from build123d import *

# Parameters (mm, degrees)
SKETCH_1_R      = 30
EXTRUDE_1_DEPTH = 20


with BuildPart() as part:
    # 草图1 → 凸台-拉伸1 (new body)
    with BuildSketch(Plane.XY):
        Circle(SKETCH_1_R)
        with BuildLine():
            Line((-3.088645972, 2.69634309), (-2.908227328, -2.89001969))
            ThreePointArc((-2.908227328, -2.89001969), (4.097863422, 0.132345676), (-3.088645972, 2.69634309))
        make_face(mode=Mode.SUBTRACT)
        with BuildLine():
            Line((22.596573624, 14.778188672), (6.935213074, 5.736097943))
            ThreePointArc((6.935213074, 5.736097943), (4.5, 7.794228634), (1.5, 8.874119675))
            Line((1.5, 8.874119675), (1.5, 26.958301133))
            ThreePointArc((1.5, 26.958301133), (13.5, 23.382685902), (22.596573624, 14.778188672))
        make_face(mode=Mode.SUBTRACT)
        with BuildLine():
            Line((-1.5, 26.958301133), (-1.5, 8.874119675))
            ThreePointArc((-1.5, 8.874119675), (-4.5, 7.794228634), (-6.935213074, 5.736097943))
            Line((-6.935213074, 5.736097943), (-22.596573624, 14.778188672))
            ThreePointArc((-22.596573624, 14.778188672), (-13.5, 23.382685902), (-1.5, 26.958301133))
        make_face(mode=Mode.SUBTRACT)
        with BuildLine():
            Line((24.096573624, 12.180112461), (8.435213074, 3.138021732))
            ThreePointArc((8.435213074, 3.138021732), (9, 0), (8.435213074, -3.138021732))
            Line((8.435213074, -3.138021732), (24.096573624, -12.180112461))
            ThreePointArc((24.096573624, -12.180112461), (27, 0), (24.096573624, 12.180112461))
        make_face(mode=Mode.SUBTRACT)
        with BuildLine():
            Line((22.596573624, -14.778188672), (6.935213074, -5.736097943))
            ThreePointArc((6.935213074, -5.736097943), (4.5, -7.794228634), (1.5, -8.874119675))
            Line((1.5, -8.874119675), (1.5, -26.958301133))
            ThreePointArc((1.5, -26.958301133), (13.5, -23.382685902), (22.596573624, -14.778188672))
        make_face(mode=Mode.SUBTRACT)
        with BuildLine():
            Line((-1.5, -26.958301133), (-1.5, -8.874119675))
            ThreePointArc((-1.5, -8.874119675), (-4.5, -7.794228634), (-6.935213074, -5.736097943))
            Line((-6.935213074, -5.736097943), (-22.596573624, -14.778188672))
            ThreePointArc((-22.596573624, -14.778188672), (-13.5, -23.382685902), (-1.5, -26.958301133))
        make_face(mode=Mode.SUBTRACT)
        with BuildLine():
            Line((-24.096573624, -12.180112461), (-8.435213074, -3.138021732))
            ThreePointArc((-8.435213074, -3.138021732), (-9, 0), (-8.435213074, 3.138021732))
            Line((-8.435213074, 3.138021732), (-24.096573624, 12.180112461))
            ThreePointArc((-24.096573624, 12.180112461), (-27, 0), (-24.096573624, -12.180112461))
        make_face(mode=Mode.SUBTRACT)
    extrude(amount=EXTRUDE_1_DEPTH)

    # 草图2 → 旋转1 (revolve)
    with BuildSketch(Plane.ZY, mode=Mode.PRIVATE) as revolve_1_sk:
        Polygon((0, -30), (0, -33), (1.6, -33), (3, -30), align=None)
        Polygon((17, -30), (20, -30), (20, -33), (18.4, -33), align=None)
        Polygon((7.8, -30), (9.2, -33), (10.8, -33), (12.2, -30), align=None)
    revolve(revolve_1_sk.sketch.rotate(Axis((0, 0, 0), (0, 0, 1)), 270), axis=Axis((0, 0, 0), (0, 0, 1)))


solid = part.part
Geometry check sheet. Reference: the model listing, model coordinates, mm. A direction names the side the tool comes from. Give positions to 0.01 mm unless a question says otherwise; leave off trailing zeros. Order: outer loops, then holes, each group sorted by start corner. A loop starts at its lowest first (then second) coordinate and runs counter-clockwise, first axis right, second up. Notation, with made-up numbers: M 88.5,24 L 116.5,24 A18 cw 116.5,45 Z; hole C -25.75,11.5 d8. An arc over 180 degrees is marked long. Use a Markdown table: item, result.
Item 1: Section check B-B (x = 0). Record the cut outline in (y, z).
Answers follow:
| item | result |
|---|---|
| outline | M -33,0 L -4.1,0 L -4.1,20 L -33,20 L -33,18.4 L -30,17 L -30,12.2 L -33,10.8 L -33,9.2 L -30,7.8 L -30,3 L -33,1.6 Z; M 4.1,0 L 33,0 L 33,1.6 L 30,3 L 30,7.8 L 33,9.2 L 33,10.8 L 30,12.2 L 30,17 L 33,18.4 L 33,20 L 4.1,20 Z |
Item 2: Depth check by flat-ended pin: P1, Ø5.5, axis at y = 14, z = 11, coming from the -X side; P2, Ø1.5, axis at y = -7.5, z = 7.5, coming from the -X side; P3, Ø5, axis at x = -16.5, z = 12.5, coming from the -Y side. Enter the tip coordinate at first touch or a pass-through.
Answers follow:
| item | result |
|---|---|
| P1 | stops at x = -31.02 |
| P2 | stops at x = -30.05 |
| P3 | stops at y = -29.56 |
Item 3: Section check A-A (z = 13.75). Record the cut outline in (x, y), and give its area (3 significant figures).
Answers follow:
| item | result |
|---|---|
| outline | C 0,0 d60; hole M -24.1,-12.18 L -8.44,-3.14 A9 cw -8.44,3.14 L -24.1,12.18 A27 ccw Z; hole M -22.6,-14.78 A27 ccw -1.5,-26.96 L -1.5,-8.87 A9 cw -6.94,-5.74 Z; hole M -22.6,14.78 L -6.94,5.74 A9 cw -1.5,8.87 L -1.5,26.96 A27 ccw Z; hole M -3.09,2.7 L -2.91,-2.89 A4.1 ccw long Z; hole M 1.5,-26.96 A27 ccw 22.6,-14.78 L 6.94,-5.74 A9 cw 1.5,-8.87 Z; hole M 1.5,8.87 A9 cw 6.94,5.74 L 22.6,14.78 A27 ccw 1.5,26.96 Z; hole M 8.44,-3.14 L 24.1,-12.18 A27 ccw 24.1,12.18 L 8.44,3.14 A9 cw Z |
| area | 1,070 mm2 |
Item 4: Draft check along X on faces 3 (the cylindrical face through (7.154, 32.215, 0.811)), 4 (the flat face through (14.876, 10.32, 9.86)), 5 (the flat face through (0, -7, 20)). Enter one of: +X half, -X half, draft (parallel to the pull), parting line (faces both ways), or undercut.
Answers follow:
| item | result |
|---|---|
| face 3 | parting line |
| face 4 | undercut |
| face 5 | draft |
Item 5: Material ranges on line 1 along Y through (x, z) = (-18, 6); line 2 along X through (y, z) = (-22.5, 14.5); line 3 along Y through (x, z) = (15, 9), recorded low to high.
Answers follow:
| item | result |
|---|---|
| line 1 | y = -24 to -20.12, -12.12 to -8.66, 8.66 to 12.12, 20.12 to 24 |
| line 2 | x = -19.84 to -14.92, -1.5 to 1.5, 14.92 to 19.84 |
| line 3 | y = -28.91 to -22.45, -10.39 to -6.93, 6.93 to 10.39, 22.45 to 28.91 |
Item 6: Tool access check on faces 1 (the flat face through (14.876, -10.32, 9.86)), 2 (the conical face through (-28.754, -9.055, 17.068)). Record the directions out of +Z, -Z, +X, -X, +Y, -Y that give a thin tool (end or side, any length) a straight path to the whole face; none if there is none.
Answers follow:
| item | result |
|---|---|
| face 1 | +Z, -Z |
| face 2 | none |
Item 7: Section check C-C (y = 0). State how many separate pieces and enclosed holes the cut face has, and give its area (3 significant figures).
Answers follow:
| item | result |
|---|---|
| separate pieces | 4 |
| enclosed holes | 0 |
| area | 384 mm2 |
